Can you work these out from the model? Positions are in its coordinate system, mm. Face numbers are marked on the shaded views. A direction names the side the tool comes from. Give positions to 0.01 mm unless a question says otherwise; leave off trailing zeros. Loops run counter-clockwise (first coordinate to the right, second up) from the corner with the lowest first, then second, coordinate; pieces in that order, holes last. Notation, with made-up numbers: M 29.25,1 L 85.25,1 A25 ccw 85.25,24 Z; hole C -31.5,-27.75 d2. An arc over 180 degrees is marked long. Use CSV: the item, a comma, the result in double quotes.
from build123d import *

# Parameters (mm, degrees)
F0_R      = 53.9289820513
F2_R      = 19.024246495
F3_FACE_R = 19.024246495
F5_R      = 54.1030648608
F7_T      = -2.54


with BuildPart() as f3:
    # F0 (on Top) → F3 section 0
    with BuildSketch(Plane.XY):
        Circle(F0_R)
    # F2 (on offset) → F3 section 1
    with BuildSketch(Plane.XY.offset(152.4)):
        Circle(F2_R)
    loft()

    # F3_face (on face) → F6 section 0
    with BuildSketch(Plane.XY.offset(152.4)):
        Circle(F3_FACE_R)
    # F5 (on offset) → F6 section 1
    with BuildSketch(Plane.XY.offset(304.8)):
        Circle(F5_R)
    loft()

    # F7
    f7_openings = [f3.faces().sort_by_distance(p)[0] for p in [
        (0, 0, 304.8),
        (0, 0, 0),
    ]]
    offset(amount=F7_T, openings=f7_openings, kind=Kind.INTERSECTION)


solid = f3.part
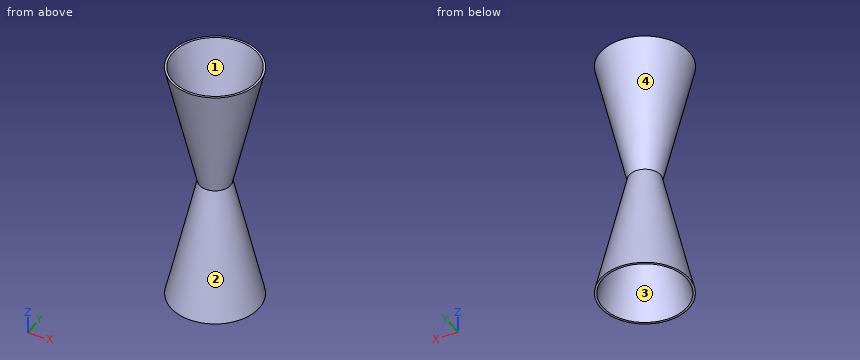
Q1. I'm going to push flat-ended pins straight in: P1, Ø5, axis at y = -27.5, z = 218, coming from the +X side; P2, Ø5, axis at x = 0.5, z = 189, coming from the -Y side; P3, Ø6, axis at x = -27, z = 87, coming from the +Y side. Where does each tip first touch, or does it pass through?
Model answer:
P1,"x = 23.36"
P2,"y = -28.02"
P3,"y = 24.24"
Q2. I want a section at B-B, the plane z = 214.5. Please give me the cut outline in (x, y).
Model answer:
outline,"C 0,0 d66.64; hole C 0,0 d61.42"
Q3. For the marked faces 3 and 4, which set-ups out of +Z, -Z, +X, -X, +Y, -Y let a thin tool reach every point of the face, with its end or its side?
Model answer:
face 3,"-Z"
face 4,"none"
Q4. I want a section at C-C, the plane z = 175. Please give me the cut outline in (x, y), then the cut area to 3 significant figures.
Model answer:
outline,"C 0,0 d48.45; hole C 0,0 d43.24"
area,"375 mm2"
Q5. Please list where these lines run through material, in increasing order: L1, parallel to Y at x = 19, z = 107.5; L2, parallel to Y at x = -3.5, z = 14; L3, parallel to X at y = 35, z = 46. Write a range as from..to.
Model answer:
L1,"-22.31..-18.76, 18.76..22.31"
L2,"-50.6..-47.99, 47.99..50.6"
L3,"-25.65..-20.94, 20.94..25.65"
Q6. I want a section at A-A, the plane x = 0. Please give me the cut outline in (y, z).
Model answer:
outline,"M -54.1,304.8 L -19.02,152.4 L -53.93,0 L -51.32,0 L -16.42,152.4 L -51.5,304.8 Z; M 16.42,152.4 L 51.32,0 L 53.93,0 L 19.02,152.4 L 54.1,304.8 L 51.5,304.8 Z"
Q7. If we mould it in two halves opening along X, with no side actions, what happens to the marked faces 1 and 2? For each: released by +X, released by -X, zero draft, split by the parting line, or undercut.
Model answer:
face 1,"undercut"
face 2,"split by the parting line"
